Design review of the part built by this model. Coordinates are the model's own, in mm. Give positions to 0.01 mm unless a question says otherwise; leave off trailing zeros. Order: outer loops, then holes, each group sorted by start corner. A loop starts at its lowest first (then second) coordinate and runs counter-clockwise, first axis right, second up. Notation, with made-up numbers: M 50.5,43.5 L 65.5,43.5 A26 cw 65.5,79.5 Z; hole C 2.25,50 d5. An arc over 180 degrees is marked long. Answer as a JSON object with one key per item and string values.
from build123d import *

# Parameters (mm, degrees)
SKETCH_1_R      = 21
SKETCH_1_R_2    = 1.5
EXTRUDE_1_DEPTH = 10
SKETCH_2_R      = 3.5
EXTRUDE_2_DEPTH = 5


with BuildPart() as part:
    # 草图1 → 凸台-拉伸1 (new body)
    with BuildSketch(Plane(origin=(0, 0, 0), x_dir=(1, 0, 0), z_dir=(0, 1, 0))):
        Circle(SKETCH_1_R)
        with Locations((-6.5, 0)):
            Circle(SKETCH_1_R_2, mode=Mode.SUBTRACT)
        with Locations((6.5, 0)):
            Circle(SKETCH_1_R_2, mode=Mode.SUBTRACT)
    extrude(amount=EXTRUDE_1_DEPTH)

    # 草图2 → 凸台-拉伸2 (add)
    with BuildSketch(Plane(origin=(0, 10, 0), x_dir=(1, 0, 0), z_dir=(0, 1, 0))):
        Circle(SKETCH_2_R)
    extrude(amount=EXTRUDE_2_DEPTH)


solid = part.part
(1) We need section D-D (x = -6.5). Write out the cut boundary in (y, z).
Checked values:
{"outline": "M 0,-19.97 L 10,-19.97 L 10,-1.5 L 0,-1.5 Z; M 0,1.5 L 10,1.5 L 10,19.97 L 0,19.97 Z"}
(2) We need section B-B (y = 8.5). Write out the cut boundary in (x, z).
Checked values:
{"outline": "C 0,0 d42; hole C -6.5,0 d3; hole C 6.5,0 d3"}
(3) To check wall thickness, follow L1, parallel to X at y = 6.5, z = 0; L2, parallel to Y at x = 5, z = -13; L3, parallel to Z at x = -7, y = 5. State the ranges of each line that lie inside material, in increasing order. Write a range as from..to.
Checked values:
{"L1": "x = -21..-8, -5..5, 8..21", "L2": "y = 0..10", "L3": "z = -19.8..-1.41, 1.41..19.8"}
(4) We need section A-A (z = 0). Write out the cut boundary in (x, y), plus the area to 3 significant figures.
Checked values:
{"outline": "M -21,0 L -8,0 L -8,10 L -21,10 Z; M -5,0 L 5,0 L 5,10 L 3.5,10 L 3.5,15 L -3.5,15 L -3.5,10 L -5,10 Z; M 8,0 L 21,0 L 21,10 L 8,10 Z", "area": "395 mm^2"}
(5) Draft analysis for pull direction Z (two halves, no side actions). For faces 1 (the cylindrical face through (3.233, 12.465, 1.341)), 2 (the flat face through (4, 10, 0)), 3 (the cylindrical face through (-8, 5, 0)), state which applies: +Z half, -Z half, draft (parallel to the pull), parting line (faces both ways), or undercut.
Checked values:
{"face 1": "parting line", "face 2": "draft", "face 3": "undercut"}
(6) We need section C-C (x = 0). Write out the cut boundary in (y, z).
Checked values:
{"outline": "M 0,-21 L 10,-21 L 10,-3.5 L 15,-3.5 L 15,3.5 L 10,3.5 L 10,21 L 0,21 Z"}
(7) Insertion check: pin 1 (6 mm diameter, centred on y = 4.5, z = -8, fed in from -X); pin 2 (2.5 mm diameter, centred on x = -6.5, z = 0, fed in from -Y); pin 3 (1.5 mm diameter, centred on x = -16, y = 3, fed in from +Z); pin 4 (10 mm diameter, centred on x = 10.5, z = 16.5, fed in from +Y). Each pin has a flat end and moves straight along its axis. Give the tip position at first contact, or say it passes through.
Checked values:
{"pin 1": "stops at x = -20.4", "pin 2": "passes through", "pin 3": "stops at z = 14.44", "pin 4": "stops at y = 10"}
